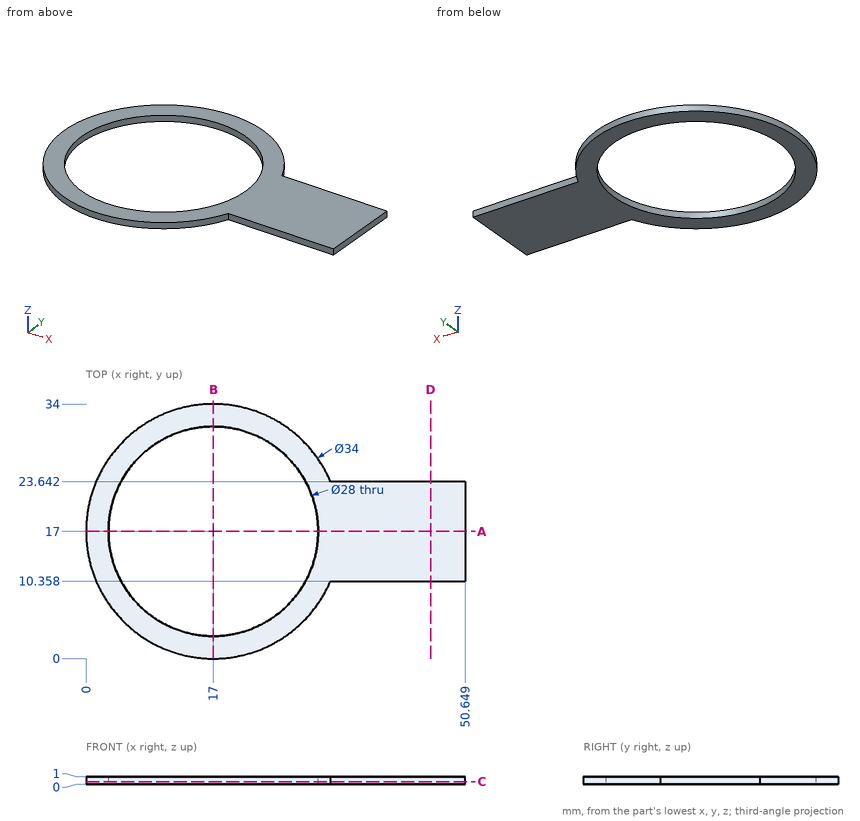
Can you work these out from the drawing? Everything is in mm from the part's minimum corner. Give positions to 0.01 mm unless a question says otherwise; leave off trailing zeros. Write each loop counter-clockwise with the first axis right and the second up, starting at its lowest first coordinate (ties: lowest second). Pieces come first, ordered by that corner, then holes. Notation, with made-up numbers: M -3.75,35.25 L 15.25,35.25 A20 cw 15.25,41.25 Z; hole C -31.5,41.5 d2. An arc over 180 degrees is marked long. Answer in a Markdown table with one row per item. Add a question column.
Item 1: Imagine slicing it at C-C, the plane z = 0.35. Write out the boundary of the cut face in (x, y), plus the area to 3 significant figures.
Item 2: Imagine slicing it at B-B, the plane x = 17. Write out the boundary of the cut face in (y, z).
Item 3: Please list where these lines run through material, in increasing order: L1, parallel to Y at x = 17, z = 0.45; L2, parallel to Y at x = 44.5, z = 0.8; L3, parallel to Y at x = 6, z = 0.55.
Item 4: Imagine slicing it at D-D, the plane x = 46. Write out the boundary of the cut face in (y, z), plus the area to 3 significant figures.
Item 5: Imagine slicing it at A-A, the plane y = 17. Write out the boundary of the cut face in (x, z).
Evaluation:
| question | item | result |
|---|---|---|
| 1 | outline | M 32.65,10.36 L 50.65,10.36 L 50.65,23.64 L 32.65,23.64 A17 ccw long Z; hole C 17,17 d28 |
| 1 | area | 519 mm² |
| 2 | outline | M 0,0 L 3,0 L 3,1 L 0,1 Z; M 31,0 L 34,0 L 34,1 L 31,1 Z |
| 3 | L1 | y = 0 to 3, 31 to 34 |
| 3 | L2 | y = 10.36 to 23.64 |
| 3 | L3 | y = 4.04 to 8.34, 25.66 to 29.96 |
| 4 | outline | M 10.36,0 L 23.64,0 L 23.64,1 L 10.36,1 Z |
| 4 | area | 13.3 mm² |
| 5 | outline | M 0,0 L 3,0 L 3,1 L 0,1 Z; M 31,0 L 50.65,0 L 50.65,1 L 31,1 Z |
